Geometry: final body of the model. Coordinates: model frame, mm. A direction names the side the tool comes from. Give positions to 0.01 mm unless a question says otherwise; leave off trailing zeros. Write each loop counter-clockwise with the first axis right and the second up, starting at its lowest first coordinate (ties: lowest second). Pieces come first, ordered by that corner, then holes. Notation, with made-up numbers: M 44.5,57.25 L 87.5,57.25 A34 cw 87.5,94.25 Z; hole C 38.5,-2 d7. An arc over 180 degrees is marked long. Use a Markdown table: item, result. Add a question column.
1) Section D-D on x = 5.5. Return the cut outline in (y, z), then the cut area to 3 significant figures.
2) Section A-A on z = 2.25. Return the cut outline in (x, y), then the cut area to 3 significant figures.
3) Line query: line 1 (Y direction, x = 0, z = 1.5); line 2 (X direction, y = -5, z = 1.95); line 3 (X direction, y = 5.5, z = 2.3). Output: solid intervals per line, ascending.
4) Draft query along Y for faces 4 (the flat face through (-7.5, 0, 1)), 5 (the cylindrical face through (-0.325, 7.464, 1.479)), 6 (the flat face through (0, 16.5, 1)), 7 (the cylindrical face through (-0.325, -9.536, 1.479)). Return one class per face: +Y half, -Y half, draft (parallel to the pull), parting line (faces both ways), or undercut.
5) Pin query (flat end, axial travel): pin 1 (1 mm diameter, centred on y = -10, z = 2.5, fed in from -X); pin 2 (1.5 mm diameter, centred on y = 10.5, z = 1.5, fed in from +X); pin 3 (1.5 mm diameter, centred on x = 9, z = 1.5, fed in from -Y). Return the tip coordinate at first contact, or that it passes through.
6) Section C-C on x = 0. Return the cut outline in (y, z).
7) Set-up query: faces 1 (the flat face through (0, 0, 0)), 2 (the flat face through (7.5, 0, 1)), 3 (the flat face through (-10, 11.5, 1)). Return all of +Z, -Z, +X, -X, +Y, -Y with unobstructed straight access to the full face (end or side cutting, diameter ignored); none if empty.
8) Section B-B on y = -11. Return the cut outline in (x, z).
Autodesk Inventor part; units mm, degrees
ref_plane "YZ Plane" through (0, 0, 0) normal (1, 0, 0) x (0, 1, 0)
ref_plane "XZ Plane" through (0, 0, 0) normal (0, 1, 0) x (-1, 0, 0)
ref_plane "XY Plane" through (0, 0, 0) normal (0, 0, 1) x (1, 0, 0)
sketch "Boceto1" plane through (0, 0, 0) normal (0, 0, 1) x (1, 0, 0)
  point P0 (0, 0)
sketch "Boceto2" plane through (0, 0, 0) normal (0, 0, 1) x (1, 0, 0)
  line L0 (-12.5, 11.5) -> (-7.5, 11.5)
  circle A0 centre (0, 6) radius 1.5
  circle A1 centre (0, -11) radius 1.5
  line L1 (7.5, 11.5) -> (12.5, 11.5)
  arc A2 (12.5, 11.5) -> (7.5, 16.5) centre (7.5, 11.5) ccw
  line L2 (7.5, 16.5) -> (-7.5, 16.5)
  arc A3 (-7.5, 16.5) -> (-12.5, 11.5) centre (-7.5, 11.5) ccw
  line L3 (-7.5, 11.5) -> (-7.5, -11.5)
  arc A4 (-7.5, -11.5) -> (-2.5, -16.5) centre (-2.5, -11.5) ccw
  line L4 (-2.5, -16.5) -> (2.5, -16.5)
  arc A5 (2.5, -16.5) -> (7.5, -11.5) centre (2.5, -11.5) ccw
  line L5 (7.5, -11.5) -> (7.5, 11.5)
  point P0 (0, 0)
  point P1 (-2.5, -16.5)
  point P2 (7.5, -11.5)
extrude "Extrusión1" add sketch "Boceto2" along normal blind 3
properties part number "Motor_Support" material "MDF Tablero de fibras de densidad media"
Found:
| question | item | result |
|---|---|---|
| 1 | outline | M -15.5,0 L 16.5,0 L 16.5,3 L -15.5,3 Z |
| 1 | area | 96.0 mm² |
| 2 | outline | M -12.5,11.5 L -7.5,11.5 L -7.5,-11.5 A5 ccw -2.5,-16.5 L 2.5,-16.5 A5 ccw 7.5,-11.5 L 7.5,11.5 L 12.5,11.5 A5 ccw 7.5,16.5 L -7.5,16.5 A5 ccw Z; hole C 0,-11 d3; hole C 0,6 d3 |
| 2 | area | 509 mm² |
| 3 | line 1 | -16.5 to -12.5, -9.5 to 4.5, 7.5 to 16.5 |
| 3 | line 2 | -7.5 to 7.5 |
| 3 | line 3 | -7.5 to -1.41, 1.41 to 7.5 |
| 4 | face 4 | draft |
| 4 | face 5 | undercut |
| 4 | face 6 | +Y half |
| 4 | face 7 | undercut |
| 5 | pin 1 | x = -7.5 |
| 5 | pin 2 | x = 7.5 |
| 5 | pin 3 | y = 11.5 |
| 6 | outline | M -16.5,0 L -12.5,0 L -12.5,3 L -16.5,3 Z; M -9.5,0 L 4.5,0 L 4.5,3 L -9.5,3 Z; M 7.5,0 L 16.5,0 L 16.5,3 L 7.5,3 Z |
| 7 | face 1 | -Z, +X, -X, +Y, -Y |
| 7 | face 2 | +Z, -Z, +X, -Y |
| 7 | face 3 | +Z, -Z, -X, -Y |
| 8 | outline | M -7.5,0 L -1.5,0 L -1.5,3 L -7.5,3 Z; M 1.5,0 L 7.5,0 L 7.5,3 L 1.5,3 Z |
